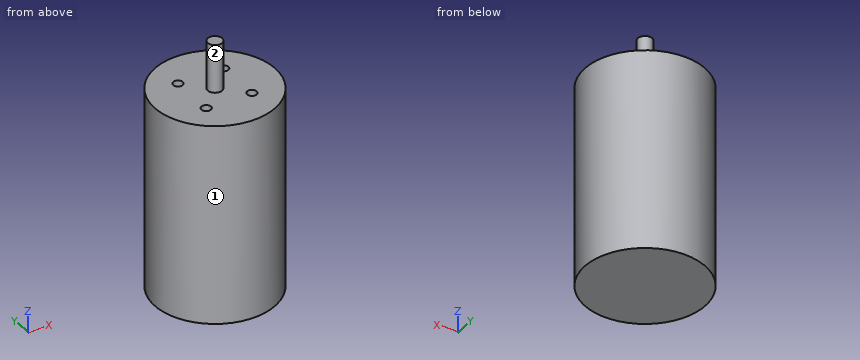
from build123d import *

# Parameters (mm, degrees)
SKETCH1_R           = 25
BOSS_EXTRUDE1_DEPTH = 83
SKETCH2_R           = 3
BOSS_EXTRUDE2_DEPTH = 20
SKETCH3_R           = 2
CUT_EXTRUDE1_DEPTH  = 10


with BuildPart() as part:
    # Sketch1 → Boss-Extrude1 (new body)
    with BuildSketch(Plane.XY):
        Circle(SKETCH1_R)
    extrude(amount=BOSS_EXTRUDE1_DEPTH)

    # Sketch2 → Boss-Extrude2 (add)
    with BuildSketch(Plane.XY.offset(83)):
        Circle(SKETCH2_R)
    extrude(amount=BOSS_EXTRUDE2_DEPTH)

    # Sketch3 → Cut-Extrude1 (cut)
    with BuildSketch(Plane.XY.offset(83)):
        with Locations((-9.5, 9.5)):
            Circle(SKETCH3_R)
        with Locations((-9.5, -9.5)):
            Circle(SKETCH3_R)
        with Locations((9.5, -9.5)):
            Circle(SKETCH3_R)
        with Locations((9.5, 9.5)):
            Circle(SKETCH3_R)
    extrude(amount=-CUT_EXTRUDE1_DEPTH, mode=Mode.SUBTRACT)


solid = part.part
Can you work these out from the model? Positions are in its coordinate system, mm. Face numbers are marked on the shaded views. A direction names the side the tool comes from. Coordinates: 2 decimals unless noted, no trailing zeros. Loops run counter-clockwise (first coordinate to the right, second up) from the corner with the lowest first, then second, coordinate; pieces in that order, holes last. Notation, with made-up numbers: M -20.5,31 L 19.5,31 A23 cw 19.5,48 Z; hole C 57.25,40.5 d11. An arc over 180 degrees is marked long. Return JSON: item names as keys, results as strings. Group by question number.
Item 1: Imagine slicing it at A-A (x = 0). Please give me the cut outline in (y, z), and give its area (3 significant figures).
Item 2: On a 3-axis mill with a long thin cutter (end or side, diameter ignored), from which of +Z, -Z, +X, -X, +Y, -Y can I reach the whole of each face in a straight line? I mean the marked faces 1 and 2. Say none if no direction works.
Item 3: Imagine slicing it at D-D (y = -9.5). Please give me the cut outline in (x, z).
Item 4: I'm going to push flat-ended pins straight in: pin 1 Ø4 at (x, z) = (-17, 13.5) entering from -Y; pin 2 Ø6 at (x, y) = (19.5, -15.5) entering from -Z; pin 3 Ø2 at (x, y) = (-9, 9) entering from +Z; pin 4 Ø4.5 at (x, y) = (-10, -10.5) entering from +Z. Where does each tip first touch, or does it pass through?
Item 5: If I drill on L1, parallel to X at y = -9, z = 76; L2, parallel to Y at x = -9.5, z = 79.25; L3, parallel to Z at x = -11, y = 7.5, over which ranges is the centre line in solid material (lowest first)? Write a range as from..to.
Item 6: Imagine slicing it at C-C (z = 36). Please give me the cut outline in (x, y).
Verdict:
{
 "1": {"outline": "M -25,0 L 25,0 L 25,83 L 3,83 L 3,103 L -3,103 L -3,83 L -25,83 Z", "area": "4,270 mm^2"},
 "2": {"face 1": "+Z, -Z", "face 2": "+Z"},
 "3": {"outline": "M -23.12,0 L 23.12,0 L 23.12,83 L 11.5,83 L 11.5,73 L 7.5,73 L 7.5,83 L -7.5,83 L -7.5,73 L -11.5,73 L -11.5,83 L -23.12,83 Z"},
 "4": {"pin 1": "stops at y = -20", "pin 2": "stops at z = 0", "pin 3": "stops at z = 73", "pin 4": "stops at z = 83"},
 "5": {"L1": "x = -23.32..-11.44, -7.56..7.56, 11.44..23.32", "L2": "y = -23.12..-11.5, -7.5..7.5, 11.5..23.12", "L3": "z = 0..83"},
 "6": {"outline": "C 0,0 d50"}
}
